Verification items for the finished model (mm, model axes). A direction names the side the tool comes from. Give positions to 0.01 mm unless a question says otherwise; leave off trailing zeros. Order: outer loops, then holes, each group sorted by start corner. A loop starts at its lowest first (then second) coordinate and runs counter-clockwise, first axis right, second up.
from build123d import *

# Parameters (mm, degrees)
SKETCH_2_W          = 80
SKETCH_2_H          = 45
EXTRUDE_1_DEPTH     = 10
EXTRUDE_2_DEPTH     = 12
FILLET_1_R          = 2
SKETCH_4_W          = 24
SKETCH_4_H          = 30
CUT_EXTRUDE_1_DEPTH = 2
SKETCH_5_W          = 28
SKETCH_5_H          = 15
EXTRUDE_3_DEPTH     = 20
CHAMFER_1_SIZE      = 5
CUT_EXTRUDE_2_DEPTH = 89.352985235
SKETCH_8_R          = 5.5
CUT_EXTRUDE_3_DEPTH = 6
SKETCH_9_R          = 3.25
CUT_EXTRUDE_4_DEPTH = 53.747037832


with BuildPart() as part:
    # 스케치2 → 보스-돌출1 (new body)
    with BuildSketch(Plane(origin=(0, 0, 0), x_dir=(1, 0, 0), z_dir=(0, 1, 0))):
        Rectangle(SKETCH_2_W, SKETCH_2_H)
    extrude(amount=EXTRUDE_1_DEPTH)

    # 스케치3 → 보스-돌출2 (add, symmetric)
    with BuildSketch(Plane(origin=(0, 0, 0), x_dir=(0, 0, -1), z_dir=(1, 0, 0))):
        Polygon((22.5, 10), (22.5, 28), (17.5, 28), (7.5, 10), align=None)
    extrude(amount=EXTRUDE_2_DEPTH, both=True)

    # 필렛1
    fillet_1_edges = [part.edges().sort_by_distance(p)[0] for p in [
        (0, 28, -22.5),
        (0, 28, -17.5),
    ]]
    fillet(fillet_1_edges, radius=FILLET_1_R)

    # 스케치4 → 컷-돌출1 (cut)
    with BuildSketch(Plane(origin=(0, 10, 0), x_dir=(1, 0, 0), z_dir=(0, 1, 0))):
        with Locations((0, -7.5)):
            Rectangle(SKETCH_4_W, SKETCH_4_H)
    extrude(amount=-CUT_EXTRUDE_1_DEPTH, mode=Mode.SUBTRACT)

    # 스케치5 → 보스-돌출3 (add)
    with BuildSketch(Plane(origin=(0, 10, 0), x_dir=(1, 0, 0), z_dir=(0, 1, 0))):
        with Locations((-26, 0.5)):
            Rectangle(SKETCH_5_W, SKETCH_5_H)
        with Locations((26, 0.5)):
            Rectangle(SKETCH_5_W, SKETCH_5_H)
    extrude(amount=EXTRUDE_3_DEPTH)

    # 모따기1
    chamfer_1_edges = [part.edges().sort_by_distance(p)[0] for p in [
        (-26, 30, 7),
        (-26, 30, -8),
        (26, 30, -8),
        (26, 30, 7),
    ]]
    chamfer(chamfer_1_edges, length=CHAMFER_1_SIZE)

    # 스케치6 → 컷-돌출2 (cut, through all)
    with BuildSketch(Plane(origin=(40, 0, 0), x_dir=(0, 0, -1), z_dir=(1, 0, 0))):
        with BuildLine():
            Line((3, 19.75), (3, 16.25))
            ThreePointArc((3, 16.25), (0.5, 13.75), (-2, 16.25))
            Line((-2, 16.25), (-2, 19.75))
            ThreePointArc((-2, 19.75), (0.5, 22.25), (3, 19.75))
        make_face()
    extrude(amount=-CUT_EXTRUDE_2_DEPTH, mode=Mode.SUBTRACT)

    # 스케치8 → 컷-돌출3 (cut)
    with BuildSketch(Plane(origin=(0, 10, 0), x_dir=(1, 0, 0), z_dir=(0, 1, 0))):
        with Locations(Location((-30, 15, 0), (0, 0, 270))):
            Circle(SKETCH_8_R)
        with Locations(Location((-30, -15, 0), (0, 0, 270))):
            Circle(SKETCH_8_R)
        with Locations(Location((30, -15, 0), (0, 0, 270))):
            Circle(SKETCH_8_R)
        with Locations(Location((30, 15, 0), (0, 0, 270))):
            Circle(SKETCH_8_R)
    extrude(amount=-CUT_EXTRUDE_3_DEPTH, mode=Mode.SUBTRACT)

    # 스케치9 → 컷-돌출4 (cut, through all)
    with BuildSketch(Plane(origin=(0, 4, 0), x_dir=(1, 0, 0), z_dir=(0, 1, 0))):
        with Locations(Location((-30, 15, 0), (0, 0, 270))):
            Circle(SKETCH_9_R)
        with Locations(Location((30, 15, 0), (0, 0, 270))):
            Circle(SKETCH_9_R)
        with Locations(Location((30, -15, 0), (0, 0, 270))):
            Circle(SKETCH_9_R)
        with Locations(Location((-30, -15, 0), (0, 0, 270))):
            Circle(SKETCH_9_R)
    extrude(amount=-CUT_EXTRUDE_4_DEPTH, mode=Mode.SUBTRACT)


solid = part.part
(1) Scan lines: line 1 (X direction, y = 2.6, z = 15); line 2 (X direction, y = 6.6, z = 15); line 3 (X direction, y = 8.2, z = 15). Record each from-to range of solid material in increasing order.
Solved:
line 1: x = -40 to -33.25, -26.75 to 26.75, 33.25 to 40
line 2: x = -40 to -35.5, -24.5 to 24.5, 35.5 to 40
line 3: x = -40 to -35.5, -24.5 to -12, 12 to 24.5, 35.5 to 40
(2) Section check B-B, the plane z = -15. Enter the section's corners in (x, y), then the cut area to 3 significant figures.
Solved:
outline: (-40, 0) - (-33.25, 0) - (-33.25, 4) - (-35.5, 4) - (-35.5, 10) - (-40, 10) - close; (-26.75, 0) - (26.75, 0) - (26.75, 4) - (24.5, 4) - (24.5, 10) - (12, 10) - (12, 23.5) - (-12, 23.5) - (-12, 10) - (-24.5, 10) - (-24.5, 4) - (-26.75, 4) - close; (33.25, 0) - (40, 0) - (40, 10) - (35.5, 10) - (35.5, 4) - (33.25, 4) - close
area: 940 mm2
(3) Go/stop test with flat-tipped pins: pin 1 (8 mm diameter, centred on x = 29.5, z = -14.5, fed in from +Y); pin 2 (1.6 mm diameter, centred on x = -4.5, y = 9.5, fed in from +Z); pin 3 (4.5 mm diameter, centred on x = 21, y = 15, fed in from +Z); pin 4 (4 mm diameter, centred on x = -30, z = -15, fed in from -Y). Record where each tip stops, or that it passes through.
Solved:
pin 1: stops at y = 4
pin 2: stops at z = -7.5
pin 3: stops at z = 7
pin 4: passes through
(4) Set-up check for faces 4 (the flat face through (-34, 4, -15)), 5 (the flat face through (12, 17, 4)), 6 (the cylindrical face through (26.827, 2.028, -15.705)), 7 (the cylindrical face through (26.2, 22.25, -0.45)): record each of +Z, -Z, +X, -X, +Y, -Y from which the full face is reachable in a straight line by a thin tool's end or side.
Solved:
face 4: +Y
face 5: +Z, +Y
face 6: +Y, -Y
face 7: +X, -X
(5) Release check for a two-part mould opening along X. For faces 1 (the flat face through (40, 11, 0)), 2 (the flat face through (-1, 10, -22.5)), 3 (the flat face through (26, 4, 15)) record: pulls with the +X half, pulls with the -X half, needs draft (parallel to the pull), parting line crosses it, or undercut.
Solved:
face 1: pulls with the +X half
face 2: needs draft
face 3: undercut
(6) Section check C-C, the plane y = 23.25. Enter the section's corners in (x, z).
Solved:
outline: (-40, -8) - (-12, -8) - (-12, 7) - (-40, 7) - close; (-12, -22.5) - (12, -22.5) - (12, -14.86) - (-12, -14.86) - close; (12, -8) - (40, -8) - (40, 7) - (12, 7) - close
(7) Section check D-D, the plane z = 3. Enter the section's corners in (x, y), then the cut area to 3 significant figures.
Solved:
outline: (-40, 0) - (40, 0) - (40, 29) - (12, 29) - (12, 8) - (-12, 8) - (-12, 29) - (-40, 29) - close
area: 1,820 mm2
(8) Section check A-A, the plane x = 30. Give the number of separate pieces and of enclosed holes in the cut face, then the cut area to 3 significant figures.
Solved:
separate pieces: 3
enclosed holes: 1
area: 504 mm2
